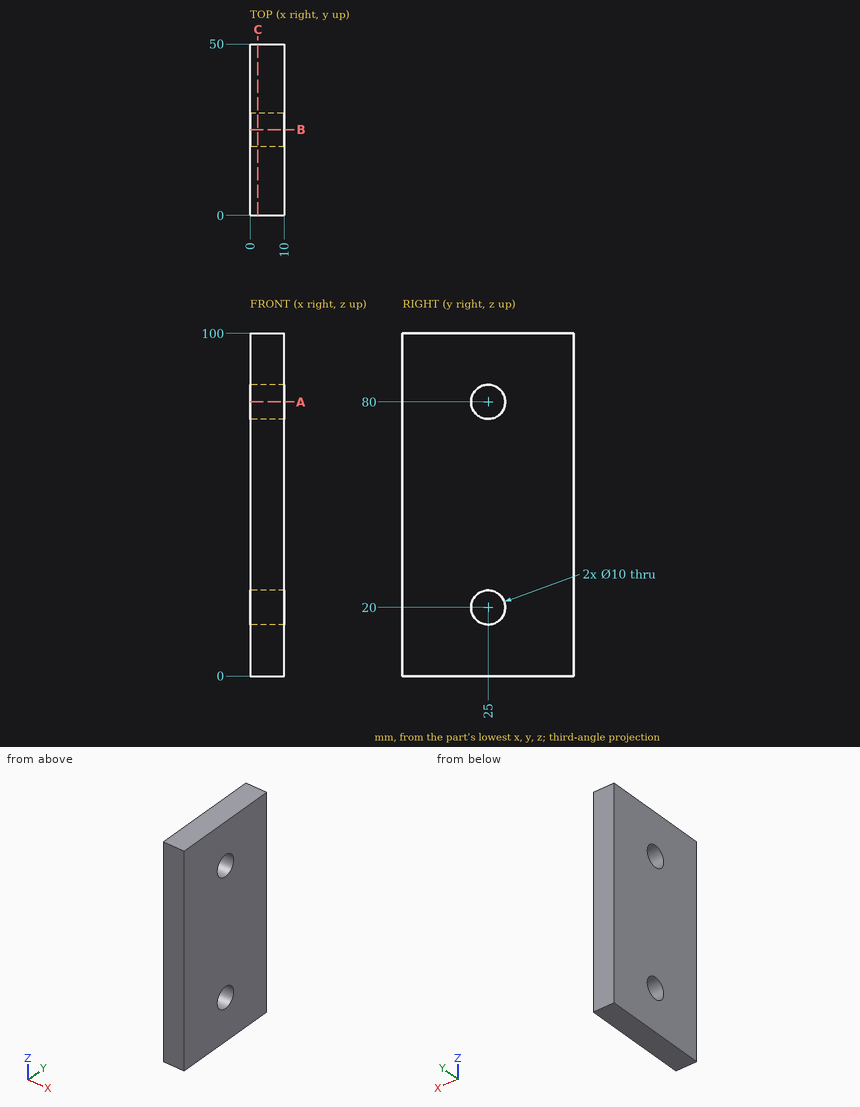
Can you work these out from the drawing? Everything is in mm from the part's minimum corner. Give positions to 0.01 mm unless a question says otherwise; leave off trailing zeros. Order: outer loops, then holes, each group sorted by start corner. A loop starts at its lowest first (then second) coordinate and runs counter-clockwise, first axis right, second up. Notation, with made-up numbers: M 1.5,30 L 59.5,30 A37 ccw 59.5,68 Z; hole C -35.5,-36 d6. An arc over 180 degrees is marked long. Use a Markdown table: item, result. Add a question column.
1. I need wall thicknesses on probe 1 along Z at (x, y) = (5.5, 25); probe 2 along Y at (x, z) = (8, 20); probe 3 along Z at (x, y) = (2.5, 24). Which ranges of each line are inside material? Lowest first, please. Write a range as from..to.
2. Suppose I cut it at B-B (y = 25). List the corners of the cut face in (x, z) for me, and give its area (3 significant figures).
3. Suppose I cut it at C-C (x = 2.25). List the corners of the cut face in (y, z) for me.
4. Suppose I cut it at A-A (z = 80). List the corners of the cut face in (x, y) for me, and give its area (3 significant figures).
Results list:
| question | item | result |
|---|---|---|
| 1 | probe 1 | z = 0..15, 25..75, 85..100 |
| 1 | probe 2 | y = 0..20, 30..50 |
| 1 | probe 3 | z = 0..15.1, 24.9..75.1, 84.9..100 |
| 2 | outline | M 0,0 L 10,0 L 10,15 L 0,15 Z; M 0,25 L 10,25 L 10,75 L 0,75 Z; M 0,85 L 10,85 L 10,100 L 0,100 Z |
| 2 | area | 800 mm² |
| 3 | outline | M 0,0 L 50,0 L 50,100 L 0,100 Z; hole C 25,20 d10; hole C 25,80 d10 |
| 4 | outline | M 0,0 L 10,0 L 10,20 L 0,20 Z; M 0,30 L 10,30 L 10,50 L 0,50 Z |
| 4 | area | 400 mm² |
